For this review, take the finished solid that the model builds, in its own axes (mm). Face numbers are marked on the shaded views. Round coordinates to 2 decimals unless told otherwise and drop trailing zeros. Loops run counter-clockwise (first coordinate to the right, second up) from the corner with the lowest first, then second, coordinate; pieces in that order, holes last. Notation, with made-up numbers: (59.25, 54) -> (110.25, 54) arc R18 cw to (110.25, 58) -> close; hole circle Ø8 at (65, 88.5). An arc over 180 degrees is marked (long way). Write each question's results on one line, items separated by ' | '.
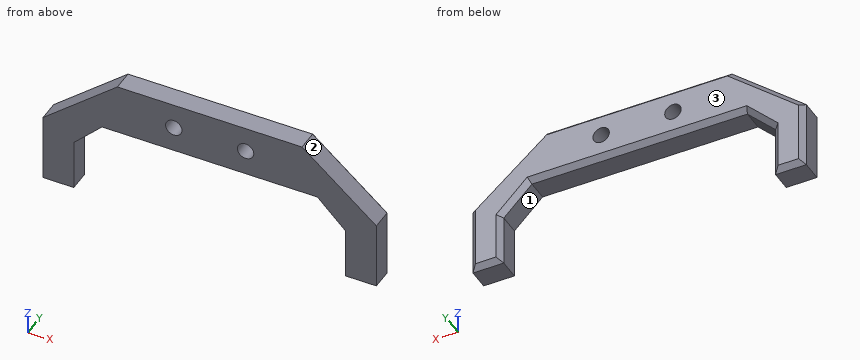
```python
from build123d import *

# Parameters (mm, degrees)
EXTRUDE_1_DEPTH     = 5
SKETCH_7_R          = 1.6
CUT_EXTRUDE_1_DEPTH = 6
CHAMFER_1_SIZE      = 1


with BuildPart() as part:
    # 草图1 → 凸台-拉伸1 (new body)
    with BuildSketch(Plane(origin=(0, 0, 0), x_dir=(1, 0, 0), z_dir=(0, 1, 0))):
        Polygon((-21, 0), (21, 0), (26.5, 5.5), (26.5, 15.5), (32.5, 15.5), (32.5, 2.166944652), (18, -10), (-18, -10), (-32.5, 2.166944652), (-32.5, 15.5), (-26.5, 15.5), (-26.5, 5.5), align=None)
    extrude(amount=EXTRUDE_1_DEPTH)

    # 草图7 → 切除-拉伸1 (cut, through all)
    with BuildSketch(Plane(origin=(0, 5, 0), x_dir=(1, 0, 0), z_dir=(0, 1, 0))):
        with Locations((-7, -5)):
            Circle(SKETCH_7_R)
        with Locations((7, -5)):
            Circle(SKETCH_7_R)
    extrude(amount=-CUT_EXTRUDE_1_DEPTH, mode=Mode.SUBTRACT)

    # 倒角1
    chamfer_1_edges = [part.edges().sort_by_distance(p)[0] for p in [
        (-23.75, 5, -2.75),
        (-26.5, 5, -10.5),
        (-29.5, 5, -15.5),
        (-32.5, 5, -8.833472326),
        (-25.25, 5, 3.916527674),
        (0, 5, 10),
        (25.25, 5, 3.916527674),
        (32.5, 5, -8.833472326),
        (29.5, 5, -15.5),
        (26.5, 5, -10.5),
        (23.75, 5, -2.75),
        (0, 5, 0),
    ]]
    chamfer(chamfer_1_edges, length=CHAMFER_1_SIZE)


solid = part.part
```
1. Consider section D-D (z = 5). State the section outline as (x, y) points, plus the area to 3 significant figures.
Values found:
outline: (-23.96, 0) -> (-8.6, 0) -> (-8.6, 5) -> (-22.4, 5) -> (-23.96, 4) -> close; (-5.4, 0) -> (5.4, 0) -> (5.4, 5) -> (-5.4, 5) -> close; (8.6, 0) -> (23.96, 0) -> (23.96, 4) -> (22.4, 5) -> (8.6, 5) -> close | area: 206 mm2
2. To check wall thickness, follow probe 1 along Z at (x, y) = (-7, 3.9); probe 2 along X at (y, z) = (1.95, 5); probe 3 along X at (y, z) = (0.9, 3.75). State the ranges of each line that lie inside material, in increasing order.
Values found:
probe 1: z = 0 to 3.4, 6.6 to 10 | probe 2: x = -23.96 to -8.6, -5.4 to 5.4, 8.6 to 23.96 | probe 3: x = -25.45 to -8, -6 to 6, 8 to 25.45
3. Consider section B-B (z = -8.25). State the section outline as (x, y) points, plus the area to 3 significant figures.
Values found:
outline: (-32.5, 0) -> (-26.5, 0) -> (-26.5, 4) -> (-27.5, 5) -> (-31.5, 5) -> (-32.5, 4) -> close; (26.5, 0) -> (32.5, 0) -> (32.5, 4) -> (31.5, 5) -> (27.5, 5) -> (26.5, 4) -> close | area: 58.0 mm2
4. For pin 1 (1.9 mm diameter, centred on x = -7, z = 5, fed in from -Y); pin 2 (3 mm diameter, centred on x = -2.5, y = 1.5, fed in from -Z), all flat-tipped, find the tip position at first contact; note any pin that passes through.
Values found:
pin 1: passes through | pin 2: stops at z = 0
5. Consider section C-C (y = 1.75). State the section outline as (x, z) points.
Values found:
outline: (-32.5, -15.5) -> (-26.5, -15.5) -> (-26.5, -5.5) -> (-21, 0) -> (21, 0) -> (26.5, -5.5) -> (26.5, -15.5) -> (32.5, -15.5) -> (32.5, -2.17) -> (18, 10) -> (-18, 10) -> (-32.5, -2.17) -> close; hole circle Ø3.2 at (-7, 5); hole circle Ø3.2 at (7, 5)
6. Consider section A-A (x = 7). State the section outline as (y, z) points, plus the area to 3 significant figures.
Values found:
outline: (0, 0) -> (4, 0) -> (5, 1) -> (5, 3.4) -> (0, 3.4) -> close; (0, 6.6) -> (5, 6.6) -> (5, 9) -> (4, 10) -> (0, 10) -> close | area: 33.0 mm2
7. Draft analysis for pull direction X (two halves, no side actions). For the marked faces 1, 2 and 3, state which applies: released by +X, released by -X, zero draft, split by the parting line, or undercut.
Values found:
face 1: undercut | face 2: released by +X | face 3: zero draft
